Geometry: final body of the model. Coordinates: model frame, mm. Give positions to 0.01 mm unless a question says otherwise; leave off trailing zeros. Order: outer loops, then holes, each group sorted by start corner. A loop starts at its lowest first (then second) coordinate and runs counter-clockwise, first axis right, second up. Notation, with made-up numbers: (30, 62) -> (74, 62) arc R23 ccw to (74, 95) -> close; hole circle Ø9 at (5, -7). An arc over 180 degrees is marked (long way). Answer in a Markdown table with one row per item. Add a question column.
Q1. Pull-direction query (Z, two-part tool) for faces 1 (the face through (-15, -11.43, 12)), 2 (the face through (-11.55, 3.13, 7.54)), 3 (the face through (-13.62, -2.66, 6.56)); classes: +Z half, -Z half, draft (parallel to the pull), parting line (faces both ways), or undercut.
Q2. Cut plane A-A on z = -42. Return the cut outline in (x, y), and give its area (3 significant figures).
Q3. Cut plane B-B on x = -61. Return the cut outline in (y, z).
Q4. Cut plane C-C on y = 3.5. Return the cut outline in (x, z).
Q5. Contact query for flat-ended pins moving along their axis: P1, Ø3, axis at x = -14.84, z = 8.91, coming from the +Y side; P2, Ø8, axis at x = -21, z = 55.5, coming from the +Y side; P3, Ø3, axis at x = -19, y = -4.5, coming from the -Z side; P4, Ø3, axis at x = 18.5, y = 0.5, coming from the +Z side. Output: stop coordinate, or through.
Q6. Line query: line 1 along Y through (x, z) = (-47.5, 32); line 2 along Z through (x, y) = (36, -0.5); line 3 along X through (y, z) = (-1.75, 54). Output: solid intervals per line, ascending. Write a range as from..to.
from build123d import *

# Parameters (mm, degrees)
F0_R     = 60.325
F1_DEPTH = 2.54
F2_R     = 3.5626601451
F3_DEPTH = 3.81
F4_DEPTH = 5.08
F5_DEPTH = 5.08
F6_R     = 2.6436042206
F7_DEPTH = 17.781


with BuildPart() as f1:
    # F0 (on Front) → F1 (new body)
    with BuildSketch(Plane.XZ):
        with Locations((-14.8387914523, 8.9064473286)):
            Circle(F0_R)
    extrude(amount=F1_DEPTH)

    # F2 (on face) → F3 (join, symmetric)
    with BuildSketch(Plane.XZ.offset(2.54)):
        with Locations((-14.8387914523, 8.9064473286)):
            Circle(F2_R)
    extrude(amount=F3_DEPTH, both=True)

    # F4 (add): a face of the model
    f4_faces = [f1.faces().sort_by_distance(p)[0] for p in [
        (-14.8387914523, 1.27, 8.9064473286),
    ]]
    extrude(f4_faces, amount=F4_DEPTH)

    # F5 (add): a face of the model
    f5_faces = [f1.faces().sort_by_distance(p)[0] for p in [
        (-14.8387914523, -6.35, 8.9064473286),
    ]]
    extrude(f5_faces, amount=F5_DEPTH)

    # F6 (on face) → F7 (cut, through all)
    with BuildSketch(Plane.XZ.offset(11.43)):
        with Locations((-14.8387914523, 8.9064473286)):
            Circle(F6_R)
    extrude(amount=-F7_DEPTH, mode=Mode.SUBTRACT)


solid = f1.part
Completed:
| question | item | result |
|---|---|---|
| 1 | face 1 | draft |
| 1 | face 2 | parting line |
| 1 | face 3 | undercut |
| 2 | outline | (-47.21, -2.54) -> (17.53, -2.54) -> (17.53, 0) -> (-47.21, 0) -> close |
| 2 | area | 164 mm² |
| 3 | outline | (-2.54, -29.93) -> (0, -29.93) -> (0, 47.74) -> (-2.54, 47.74) -> close |
| 4 | outline | circle Ø7.13 at (-14.84, 8.91); hole circle Ø5.29 at (-14.84, 8.91) |
| 5 | P1 | passes through |
| 5 | P2 | stops at y = 0 |
| 5 | P3 | stops at z = 6.54 |
| 5 | P4 | stops at z = 60.09 |
| 6 | line 1 | y = -2.54..0 |
| 6 | line 2 | z = -23.57..41.38 |
| 6 | line 3 | x = -54.91..25.23 |
